from build123d import *

# Parameters (mm, degrees)
F1_DEPTH = 25.4
F2_DEPTH = 25.4
F3_DEPTH = 25.4
F4_DEPTH = 25.4


with BuildPart() as f1:
    # F0 (on Front) → F1 (new body)
    with BuildSketch(Plane.XZ):
        with BuildLine():
            Line((34.9249988794, 38.3535841248), (34.9249988794, 9.525))
            Line((34.9249988794, 9.525), (41.275, 9.525))
            Line((41.275, 9.525), (41.275, 38.3535841248))
            ThreePointArc((41.275, 38.3535841248), (43.6085299046, 46.6387644279), (49.9230897833, 52.4882009827))
            Line((49.9230897833, 52.4882009827), (49.9230897833, 59.3707781223))
            ThreePointArc((49.9230897833, 59.3707781223), (39.0589972297, 51.2635141623), (34.9249988794, 38.3535841248))
        make_face()
        with BuildLine():
            Line((41.275, 9.525), (34.9249988794, 9.525))
            Line((34.9249988794, 9.525), (27.6167455206, 9.525))
            ThreePointArc((27.6167455206, 9.525), (28.811311946, 4.8289297054), (29.2131863745, 0))
            ThreePointArc((29.2131863745, 0), (28.811311946, -4.8289297054), (27.6167455206, -9.525))
            Line((27.6167455206, -9.525), (41.275, -9.525))
            Line((41.275, -9.525), (41.275, 9.525))
        make_face()
        with BuildLine():
            ThreePointArc((29.2131863745, 0), (28.811311946, 4.8289297054), (27.6167455206, 9.525))
            Line((27.6167455206, 9.525), (-27.6167455206, 9.525))
            ThreePointArc((-27.6167455206, 9.525), (-29.2131863745, 0), (-27.6167455206, -9.525))
            Line((-27.6167455206, -9.525), (27.6167455206, -9.525))
            ThreePointArc((27.6167455206, -9.525), (28.811311946, -4.8289297054), (29.2131863745, 0))
        make_face()
        with BuildLine():
            Line((-27.6167455206, 9.525), (27.6167455206, 9.525))
            ThreePointArc((27.6167455206, 9.525), (0, 29.2131863745), (-27.6167455206, 9.525))
        make_face()
        with BuildLine():
            ThreePointArc((-27.6167455206, -9.525), (-29.2131863745, 0), (-27.6167455206, 9.525))
            Line((-27.6167455206, 9.525), (-41.275, 9.525))
            Line((-41.275, 9.525), (-41.275, -9.525))
            Line((-41.275, -9.525), (-27.6167455206, -9.525))
        make_face()
        Polygon((49.9230897833, 71.0192042329), (49.9230897833, 59.3707781223), (49.9230897833, 52.4882009827), (49.9230897833, 26.4684122215), (100.7230897833, 26.4684122215), (100.7230897833, 71.0192042329), align=None)
        with BuildLine():
            ThreePointArc((-27.6167455206, -9.525), (0, -29.2131863745), (27.6167455206, -9.525))
            Line((27.6167455206, -9.525), (-27.6167455206, -9.525))
        make_face()
    extrude(amount=F1_DEPTH)

    # F0 (on Front) → F2 (join)
    with BuildSketch(Plane.XZ):
        with BuildLine():
            Line((34.9249988794, 38.3535841248), (34.9249988794, 9.525))
            Line((34.9249988794, 9.525), (41.275, 9.525))
            Line((41.275, 9.525), (41.275, 38.3535841248))
            ThreePointArc((41.275, 38.3535841248), (43.6085299046, 46.6387644279), (49.9230897833, 52.4882009827))
            Line((49.9230897833, 52.4882009827), (49.9230897833, 59.3707781223))
            ThreePointArc((49.9230897833, 59.3707781223), (39.0589972297, 51.2635141623), (34.9249988794, 38.3535841248))
        make_face()
        with BuildLine():
            Line((41.275, 9.525), (34.9249988794, 9.525))
            Line((34.9249988794, 9.525), (27.6167455206, 9.525))
            ThreePointArc((27.6167455206, 9.525), (28.811311946, 4.8289297054), (29.2131863745, 0))
            ThreePointArc((29.2131863745, 0), (28.811311946, -4.8289297054), (27.6167455206, -9.525))
            Line((27.6167455206, -9.525), (41.275, -9.525))
            Line((41.275, -9.525), (41.275, 9.525))
        make_face()
        with BuildLine():
            ThreePointArc((29.2131863745, 0), (28.811311946, 4.8289297054), (27.6167455206, 9.525))
            Line((27.6167455206, 9.525), (-27.6167455206, 9.525))
            ThreePointArc((-27.6167455206, 9.525), (-29.2131863745, 0), (-27.6167455206, -9.525))
            Line((-27.6167455206, -9.525), (27.6167455206, -9.525))
            ThreePointArc((27.6167455206, -9.525), (28.811311946, -4.8289297054), (29.2131863745, 0))
        make_face()
        with BuildLine():
            Line((-27.6167455206, 9.525), (27.6167455206, 9.525))
            ThreePointArc((27.6167455206, 9.525), (0, 29.2131863745), (-27.6167455206, 9.525))
        make_face()
        with BuildLine():
            ThreePointArc((-27.6167455206, -9.525), (-29.2131863745, 0), (-27.6167455206, 9.525))
            Line((-27.6167455206, 9.525), (-41.275, 9.525))
            Line((-41.275, 9.525), (-41.275, -9.525))
            Line((-41.275, -9.525), (-27.6167455206, -9.525))
        make_face()
        Polygon((49.9230897833, 71.0192042329), (49.9230897833, 59.3707781223), (49.9230897833, 52.4882009827), (49.9230897833, 26.4684122215), (100.7230897833, 26.4684122215), (100.7230897833, 71.0192042329), align=None)
        with BuildLine():
            ThreePointArc((-27.6167455206, -9.525), (0, -29.2131863745), (27.6167455206, -9.525))
            Line((27.6167455206, -9.525), (-27.6167455206, -9.525))
        make_face()
    extrude(amount=F2_DEPTH)

    # F0 (on Front) → F3 (join)
    with BuildSketch(Plane.XZ):
        with BuildLine():
            Line((34.9249988794, 38.3535841248), (34.9249988794, 9.525))
            Line((34.9249988794, 9.525), (41.275, 9.525))
            Line((41.275, 9.525), (41.275, 38.3535841248))
            ThreePointArc((41.275, 38.3535841248), (43.6085299046, 46.6387644279), (49.9230897833, 52.4882009827))
            Line((49.9230897833, 52.4882009827), (49.9230897833, 59.3707781223))
            ThreePointArc((49.9230897833, 59.3707781223), (39.0589972297, 51.2635141623), (34.9249988794, 38.3535841248))
        make_face()
        with BuildLine():
            Line((41.275, 9.525), (34.9249988794, 9.525))
            Line((34.9249988794, 9.525), (27.6167455206, 9.525))
            ThreePointArc((27.6167455206, 9.525), (28.811311946, 4.8289297054), (29.2131863745, 0))
            ThreePointArc((29.2131863745, 0), (28.811311946, -4.8289297054), (27.6167455206, -9.525))
            Line((27.6167455206, -9.525), (41.275, -9.525))
            Line((41.275, -9.525), (41.275, 9.525))
        make_face()
        with BuildLine():
            ThreePointArc((29.2131863745, 0), (28.811311946, 4.8289297054), (27.6167455206, 9.525))
            Line((27.6167455206, 9.525), (-27.6167455206, 9.525))
            ThreePointArc((-27.6167455206, 9.525), (-29.2131863745, 0), (-27.6167455206, -9.525))
            Line((-27.6167455206, -9.525), (27.6167455206, -9.525))
            ThreePointArc((27.6167455206, -9.525), (28.811311946, -4.8289297054), (29.2131863745, 0))
        make_face()
        with BuildLine():
            Line((-27.6167455206, 9.525), (27.6167455206, 9.525))
            ThreePointArc((27.6167455206, 9.525), (0, 29.2131863745), (-27.6167455206, 9.525))
        make_face()
        with BuildLine():
            ThreePointArc((-27.6167455206, -9.525), (-29.2131863745, 0), (-27.6167455206, 9.525))
            Line((-27.6167455206, 9.525), (-41.275, 9.525))
            Line((-41.275, 9.525), (-41.275, -9.525))
            Line((-41.275, -9.525), (-27.6167455206, -9.525))
        make_face()
        Polygon((49.9230897833, 71.0192042329), (49.9230897833, 59.3707781223), (49.9230897833, 52.4882009827), (49.9230897833, 26.4684122215), (100.7230897833, 26.4684122215), (100.7230897833, 71.0192042329), align=None)
        with BuildLine():
            ThreePointArc((-27.6167455206, -9.525), (0, -29.2131863745), (27.6167455206, -9.525))
            Line((27.6167455206, -9.525), (-27.6167455206, -9.525))
        make_face()
    extrude(amount=F3_DEPTH)

    # F0 (on Front) → F4 (join)
    with BuildSketch(Plane.XZ):
        with BuildLine():
            Line((34.9249988794, 38.3535841248), (34.9249988794, 9.525))
            Line((34.9249988794, 9.525), (41.275, 9.525))
            Line((41.275, 9.525), (41.275, 38.3535841248))
            ThreePointArc((41.275, 38.3535841248), (43.6085299046, 46.6387644279), (49.9230897833, 52.4882009827))
            Line((49.9230897833, 52.4882009827), (49.9230897833, 59.3707781223))
            ThreePointArc((49.9230897833, 59.3707781223), (39.0589972297, 51.2635141623), (34.9249988794, 38.3535841248))
        make_face()
        with BuildLine():
            Line((41.275, 9.525), (34.9249988794, 9.525))
            Line((34.9249988794, 9.525), (27.6167455206, 9.525))
            ThreePointArc((27.6167455206, 9.525), (28.811311946, 4.8289297054), (29.2131863745, 0))
            ThreePointArc((29.2131863745, 0), (28.811311946, -4.8289297054), (27.6167455206, -9.525))
            Line((27.6167455206, -9.525), (41.275, -9.525))
            Line((41.275, -9.525), (41.275, 9.525))
        make_face()
        with BuildLine():
            ThreePointArc((29.2131863745, 0), (28.811311946, 4.8289297054), (27.6167455206, 9.525))
            Line((27.6167455206, 9.525), (-27.6167455206, 9.525))
            ThreePointArc((-27.6167455206, 9.525), (-29.2131863745, 0), (-27.6167455206, -9.525))
            Line((-27.6167455206, -9.525), (27.6167455206, -9.525))
            ThreePointArc((27.6167455206, -9.525), (28.811311946, -4.8289297054), (29.2131863745, 0))
        make_face()
        with BuildLine():
            Line((-27.6167455206, 9.525), (27.6167455206, 9.525))
            ThreePointArc((27.6167455206, 9.525), (0, 29.2131863745), (-27.6167455206, 9.525))
        make_face()
        with BuildLine():
            ThreePointArc((-27.6167455206, -9.525), (-29.2131863745, 0), (-27.6167455206, 9.525))
            Line((-27.6167455206, 9.525), (-41.275, 9.525))
            Line((-41.275, 9.525), (-41.275, -9.525))
            Line((-41.275, -9.525), (-27.6167455206, -9.525))
        make_face()
        Polygon((49.9230897833, 71.0192042329), (49.9230897833, 59.3707781223), (49.9230897833, 52.4882009827), (49.9230897833, 26.4684122215), (100.7230897833, 26.4684122215), (100.7230897833, 71.0192042329), align=None)
        with BuildLine():
            ThreePointArc((-27.6167455206, -9.525), (0, -29.2131863745), (27.6167455206, -9.525))
            Line((27.6167455206, -9.525), (-27.6167455206, -9.525))
        make_face()
    extrude(amount=F4_DEPTH)


solid = f1.part
Verification items for the finished model (mm, model axes). A direction names the side the tool comes from. Give positions to 0.01 mm unless a question says otherwise; leave off trailing zeros. Order: outer loops, then holes, each group sorted by start corner. A loop starts at its lowest first (then second) coordinate and runs counter-clockwise, first axis right, second up. Notation, with made-up numbers: M -26,47 L 0,47 A14 cw 0,51 Z; hole C 40,-34.75 d11. An arc over 180 degrees is marked long. Answer as a JSON object with one key per item and string values. Group by question number.
1) Scan lines: line 1 along X through (y, z) = (-6, 33.5) (3 decimals); line 2 along X through (y, z) = (-18, 26.5) (3 decimals); line 3 along Z through (x, y) = (79.5, -6.5). Record each from-to range of solid material in increasing order. Write a range as [from, to].
2) Cross-section at A-A (z = 43). Enter the section's corners in (x, y), then the cut area to 3 significant figures.
3) Cross-section at B-B (y = -2). Enter the section's corners in (x, z) (3 decimals).
4) Cross-section at C-C (z = 61). Enter the section's corners in (x, y), then the cut area to 3 significant figures.
5) Access from +Z, -Z, +X, -X, +Y, -Y to the whole of each face (thin tool, end or side, straight path). Record for faces 1 (the face through (41.275, -13, 14)), 2 (the face through (75, -13, 26.468)), 3 (the face through (-35, -13, -9.525)), 4 (the face through (49.923, -13, 65)).
6) Cross-section at D-D (x = 33). Enter the section's corners in (y, z) (3 decimals), then the cut area to 3 significant figures.
7) Depth check by flat-ended pin: pin 1 Ø3 at (x, y) = (65, -23) entering from -Z; pin 2 Ø7.5 at (y, z) = (-7, 20) entering from -X; pin 3 Ø7.5 at (y, z) = (-14.5, 33.5) entering from -X (3 decimals); pin 4 Ø10 at (x, z) = (67, 21.5) entering from -Y. Enter the tip coordinate at first touch or a pass-through.
8) Mould release check, pull along X, two halves, no side actions. Record for faces 5 (the face through (31, -13, 9.525)), 6 (the face through (34, -13, -9.525)), 7 (the face through (-41.275, -13, 0)), 8 (the face through (100.723, -13, 48)): released by +X, released by -X, zero draft, split by the parting line, or undercut.
Result sheet:
{
 "1": {"line 1": "x = [34.925, 41.275], [49.923, 100.723]", "line 2": "x = [-12.295, 12.295], [34.925, 41.275], [49.923, 100.723]", "line 3": "z = [26.47, 71.02]"},
 "2": {"outline": "M 35.42,-25.4 L 41.97,-25.4 L 41.97,0 L 35.42,0 Z; M 49.92,-25.4 L 100.72,-25.4 L 100.72,0 L 49.92,0 Z", "area": "1,460 mm2"},
 "3": {"outline": "M -41.275,-9.525 L -27.617,-9.525 A29.213 ccw 27.617,-9.525 L 41.275,-9.525 L 41.275,38.354 A15.875 cw 49.923,52.488 L 49.923,26.468 L 100.723,26.468 L 100.723,71.019 L 49.923,71.019 L 49.923,59.371 A22.225 ccw 34.925,38.354 L 34.925,9.525 L 27.617,9.525 A29.213 ccw -27.617,9.525 L -41.275,9.525 Z"},
 "4": {"outline": "M 49.92,-25.4 L 100.72,-25.4 L 100.72,0 L 49.92,0 Z", "area": "1,290 mm2"},
 "5": {"face 1": "-Z, +Y, -Y", "face 2": "-Z, +X, +Y, -Y", "face 3": "-Z, -X, +Y, -Y", "face 4": "+Z, -X, +Y, -Y"},
 "6": {"outline": "M -25.4,-9.525 L 0,-9.525 L 0,9.525 L -25.4,9.525 Z", "area": "484 mm2"},
 "7": {"pin 1": "stops at z = 26.47", "pin 2": "stops at x = -24.28", "pin 3": "stops at x = 34.925", "pin 4": "stops at y = -25.4"},
 "8": {"face 5": "undercut", "face 6": "zero draft", "face 7": "released by -X", "face 8": "released by +X"}
}
